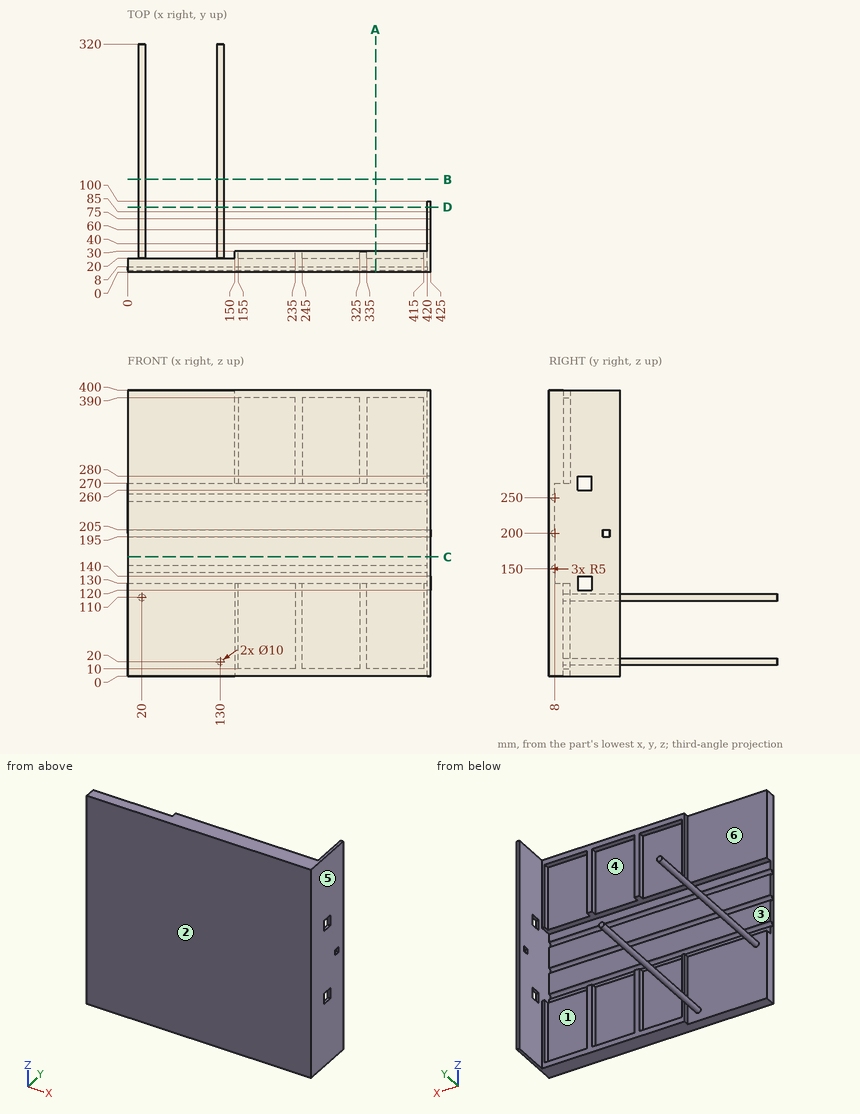
The figure shows three views and two pictorial views of one solid part (mm, origin at its lowest corner). Answer the questions. A direction names the side the tool comes from. Coordinates: 2 decimals unless noted, no trailing zeros. Order: outer loops, then holes, each group sorted by start corner. A loop starts at its lowest first (then second) coordinate and runs counter-clockwise, first axis right, second up.
Q1. Given P1, Ø5, axis at x = 132.5, y = 49.5, coming from the +Z side; P2, Ø24, axis at x = 209.5, z = 352, coming from the +Y side; P3, Ø8, axis at y = 26.5, z = 83.5, coming from the -X side, each flat-ended and moving along its own axis, determine where each tip first touches the part or whether it passes through.
Q2. A cutting plane is placed at B-B, the plane y = 130.5. Write down the section's boundary in (x, z), and give its area (3 significant figures).
Q3. A cutting plane is placed at C-C, the plane z = 167. Write down the section's boundary in (x, y), and give its area (3 significant figures).
Q4. A cutting plane is placed at D-D, the plane y = 91.5. Write down the section's boundary in (x, z), and give its area (3 significant figures).
Q5. A cutting plane is placed at A-A, the plane x = 347.5. Write down the section's boundary in (y, z).
Q6. Consider line 1 (X direction, y = 22, z = 350); line 2 (Y direction, x = 151, z = 332); line 3 (Y direction, x = 71, z = 345.5). Determine where each line is inside the solid, lowest interval first.
Q7. For a pull along X with two mould halves and no side action, classify the marked faces 4, 5 and 6 as pulls with the +X half, pulls with the -X half, needs draft (parallel to the pull), parting line crosses it, or undercut.
Q8. Which of the six approach directions +Z, -Z, +X, -X, +Y, -Y give full straight-line access (tool end or side, diameter ignored) to the marked faces 1, 2 and 3?
Answers follow:
1. P1: stops at z = 25
1. P2: stops at y = 20
1. P3: stops at x = 150
2. outline: circle Ø10 at (20, 110); circle Ø10 at (130, 20)
2. area: 157 mm2
3. outline: (0, 0) - (425, 0) - (425, 100) - (420, 100) - (420, 8) - (0, 8) - close
3. area: 3,860 mm2
4. outline: circle Ø10 at (20, 110); circle Ø10 at (130, 20); (420, 0) - (425, 0) - (425, 400) - (420, 400) - close
4. area: 2,160 mm2
5. outline: (0, 0) - (30, 0) - (30, 10) - (20, 10) - (20, 130) - (8, 130) - (8, 145) arc R5 cw to (8, 155) - (8, 195) arc R5 cw to (8, 205) - (8, 245) arc R5 cw to (8, 255) - (8, 270) - (20, 270) - (20, 390) - (30, 390) - (30, 400) - (0, 400) - close
6. line 1: x = 150 to 155, 235 to 245, 325 to 335, 415 to 425
6. line 2: y = 0 to 30
6. line 3: y = 0 to 20
7. face 4: undercut
7. face 5: pulls with the +X half
7. face 6: needs draft
8. face 1: +Y
8. face 2: +Z, -Z, +X, -X, -Y
8. face 3: -X, +Y
